Source: CAD feature listing. Evaluate the final solid. Frame: model axes, mm. A direction names the side the tool comes from. Give positions to 0.01 mm unless a question says otherwise; leave off trailing zeros. Write each loop counter-clockwise with the first axis right and the second up, starting at its lowest first coordinate (ties: lowest second). Pieces come first, ordered by that corner, then holes. Notation, with made-up numbers: (63, 19) -> (119, 19) arc R15 cw to (119, 39) -> close; hole circle Ø7 at (6, -31). An arc over 180 degrees is marked (long way). Write item = value, one per line.
from build123d import *

# Parameters (mm, degrees)
SALIENTE_EXTRUIR1_DEPTH = 8
CROQUIS2_R              = 4.25
CORTAR_EXTRUIR1_DEPTH   = 9
CROQUIS3_OUTSIDE_W      = 57.674
CROQUIS3_OUTSIDE_H      = 54.734
CROQUIS3_OUTSIDE_R      = 9.5
CORTAR_EXTRUIR2_DEPTH   = 8
CORTAR_EXTRUIR2_TAPER   = 60
CROQUIS4_OUTSIDE_W      = 57.674
CROQUIS4_OUTSIDE_H      = 54.734
CROQUIS4_OUTSIDE_R      = 9.5
CORTAR_EXTRUIR3_DEPTH   = 8
CORTAR_EXTRUIR3_TAPER   = 60
CROQUIS5_R              = 5
SALIENTE_EXTRUIR3_DEPTH = 120
CHAFL_N2_SIZE           = 1


with BuildPart() as part:
    # Croquis1 → Saliente-Extruir1 (new body)
    with BuildSketch(Plane(origin=(0, 0, 0), x_dir=(1, 0, 0), z_dir=(0, 1, 0))):
        Polygon((10.969655115, 0), (5.484827557, 9.5), (-5.484827557, 9.5), (-10.969655115, 0), (-5.484827557, -9.5), (5.484827557, -9.5), align=None)
    extrude(amount=SALIENTE_EXTRUIR1_DEPTH)

    # Croquis2 → Cortar-Extruir1 (cut, through all)
    with BuildSketch(Plane(origin=(0, 8, 0), x_dir=(1, 0, 0), z_dir=(0, 1, 0))):
        Circle(CROQUIS2_R)
    extrude(amount=-CORTAR_EXTRUIR1_DEPTH, mode=Mode.SUBTRACT)

    # Croquis3 outside → Cortar-Extruir2 (cut)
    with BuildSketch(Plane(origin=(0, 8, 0), x_dir=(1, 0, 0), z_dir=(0, 1, 0))):
        Rectangle(CROQUIS3_OUTSIDE_W, CROQUIS3_OUTSIDE_H)
        Circle(CROQUIS3_OUTSIDE_R, mode=Mode.SUBTRACT)
    extrude(amount=-CORTAR_EXTRUIR2_DEPTH, taper=CORTAR_EXTRUIR2_TAPER, mode=Mode.SUBTRACT)

    # Croquis4 outside → Cortar-Extruir3 (cut)
    with BuildSketch(Plane.XZ):
        Rectangle(CROQUIS4_OUTSIDE_W, CROQUIS4_OUTSIDE_H)
        Circle(CROQUIS4_OUTSIDE_R, mode=Mode.SUBTRACT)
    extrude(amount=-CORTAR_EXTRUIR3_DEPTH, taper=CORTAR_EXTRUIR3_TAPER, mode=Mode.SUBTRACT)

    # Croquis5 → Saliente-Extruir3 (add)
    with BuildSketch(Plane(origin=(0, 8, 0), x_dir=(1, 0, 0), z_dir=(0, 1, 0))):
        Circle(CROQUIS5_R)
    extrude(amount=-SALIENTE_EXTRUIR3_DEPTH)

    # Chaflán2
    chafl_n2_edges = [part.edges().sort_by_distance(p)[0] for p in [
        (-5, -112, 0),
    ]]
    chamfer(chafl_n2_edges, length=CHAFL_N2_SIZE)


solid = part.part
(1) Access query for faces 1 (the face through (-1.08, -54.72, 4.88)), 2 (the face through (-4.908, 0.206, -8.549)). Directions: +Z, -Z, +X, -X, +Y, -Y. A direction counts if a zero-diameter tool reaches every point of the face in a straight line with its end or side. Return the directions, or none.
Values follow:
face_1 = -Y
face_2 = -Z, -X, -Y
(2) Section query A-A (y = -61.5). Return loops of the section in (x, z).
Values follow:
outline = circle Ø10 at (0, 0)
(3) Material intervals for line 1 (Y direction, x = 3.25, z = -5); line 2 (X direction, y = -31, z = -3); line 3 (X direction, y = -56, z = -1.5), sorted ascending.
Values follow:
line_1 = 0 to 8
line_2 = -4 to 4
line_3 = -4.77 to 4.77
(4) First-contact query: pin 1 (3 mm diameter, centred on y = -41.5, z = -5.5, fed in from -X); pin 2 (10 mm diameter, centred on y = -23, z = 4, fed in from -X); pin 3 (4 mm diameter, centred on x = 1, y = -73, fed in from +Z). Flat tips, straight axial feed; report the tip coordinate or a pass-through.
Values follow:
pin_1 = -3
pin_2 = -5
pin_3 = 5
